```python
from build123d import *

# Parameters (mm, degrees)
SKETCH1_W           = 5
SKETCH1_H           = 4
SKETCH1_W_2         = 3
SKETCH1_H_2         = 2
BOSS_EXTRUDE1_DEPTH = 10
SKETCH2_W           = 5
SKETCH2_H           = 4
SKETCH2_R           = 1.65
BOSS_EXTRUDE2_DEPTH = 1
SKETCH3_R           = 1.65
CUT_EXTRUDE1_DEPTH  = 12.456439237


with BuildPart() as part:
    # Sketch1 → Boss-Extrude1 (new body)
    with BuildSketch(Plane.XY):
        Rectangle(SKETCH1_W, SKETCH1_H)
        Rectangle(SKETCH1_W_2, SKETCH1_H_2, mode=Mode.SUBTRACT)
    extrude(amount=BOSS_EXTRUDE1_DEPTH)

    # Sketch2 → Boss-Extrude2 (add)
    with BuildSketch(Plane.XY.offset(10)):
        Rectangle(SKETCH2_W, SKETCH2_H)
        with Locations(Location((0, 0, 0), (0, 0, 155.380022671))):
            Circle(SKETCH2_R, mode=Mode.SUBTRACT)
    extrude(amount=BOSS_EXTRUDE2_DEPTH)

    # Sketch3 → Cut-Extrude1 (cut, through all)
    with BuildSketch(Plane.XY.offset(11)):
        with Locations(Location((0, 0, 0), (0, 0, 155.380022671))):
            Circle(SKETCH3_R)
    extrude(amount=-CUT_EXTRUDE1_DEPTH, mode=Mode.SUBTRACT)


solid = part.part
```
Read the model definition and answer for the solid it produces. Units are mm, in the model's axes. Coordinates: 2 decimals unless noted, no trailing zeros. Loops run counter-clockwise (first coordinate to the right, second up) from the corner with the lowest first, then second, coordinate; pieces in that order, holes last.
(1) The part is cut by section A-A (x = 0). Determine the outline of the cut face in (y, z), and give its area (3 significant figures).
Solution:
outline: (-2, 0) - (-1.65, 0) - (-1.65, 11) - (-2, 11) - close; (1.65, 0) - (2, 0) - (2, 11) - (1.65, 11) - close
area: 7.70 mm2
(2) Consider line 1 along Y through (x, z) = (-1.45, 0.5); line 2 along Y through (x, z) = (0, 10.2); line 3 along X through (y, z) = (0, 4.75). Determine where each line is inside the solid, lowest interval first.
Solution:
line 1: y = -2 to -1, 1 to 2
line 2: y = -2 to -1.65, 1.65 to 2
line 3: x = -2.5 to -1.65, 1.65 to 2.5
(3) The part is cut by section C-C (z = 6.5). Determine the outline of the cut face in (x, y).
Solution:
outline: (-2.5, -2) - (2.5, -2) - (2.5, 2) - (-2.5, 2) - close; hole (-1.5, -1) - (-1.31, -1) arc R1.65 ccw to (1.31, -1) - (1.5, -1) - (1.5, -0.69) arc R1.65 ccw to (1.5, 0.69) - (1.5, 1) - (1.31, 1) arc R1.65 ccw to (-1.31, 1) - (-1.5, 1) - (-1.5, 0.69) arc R1.65 ccw to (-1.5, -0.69) - close
(4) The part is cut by section B-B (y = 0). Determine the outline of the cut face in (x, z).
Solution:
outline: (-2.5, 0) - (-1.65, 0) - (-1.65, 11) - (-2.5, 11) - close; (1.65, 0) - (2.5, 0) - (2.5, 11) - (1.65, 11) - close
(5) The part is cut by section D-D (y = 0.8). Determine the outline of the cut face in (x, z).
Solution:
outline: (-2.5, 0) - (-1.5, 0) - (-1.5, 10) - (-1.44, 10) - (-1.44, 11) - (-2.5, 11) - close; (1.44, 10) - (1.5, 10) - (1.5, 0) - (2.5, 0) - (2.5, 11) - (1.44, 11) - close
